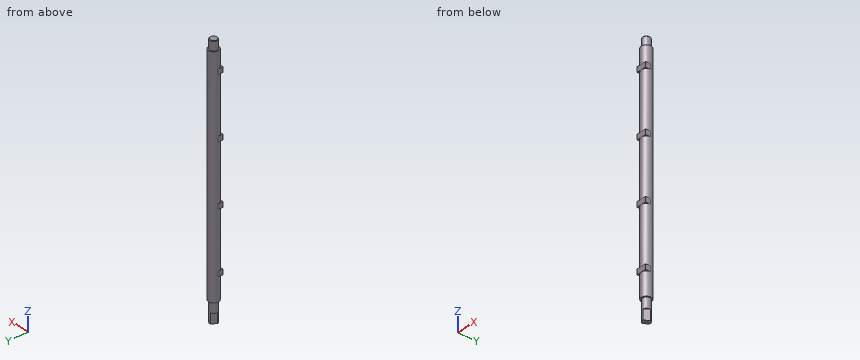
Autodesk Inventor part; units mm, degrees
ref_plane "工作平面1" through (0, 0, 45) normal (0, 0, -1) x (-1, 0, 0)
ref_plane "YZ Plane" through (0, 0, 0) normal (1, 0, 0) x (0, 1, 0)
ref_plane "XZ Plane" through (0, 0, 0) normal (0, 1, 0) x (-1, 0, 0)
sketch "草图1" plane through (0, 0, 0) normal (0, 0, 1) x (1, 0, 0)
  circle A0 centre (0, 0) radius 10
  dimension "d0" = 20
extrude "拉伸1" add sketch "草图1" along normal blind 447
sketch "草图2" plane through (0, 0, 447) normal (0, 0, 1) x (1, 0, 0)
  circle A0 centre (0, 0) radius 7.5
  dimension "d3" = 15
extrude "拉伸2" add sketch "草图2" along normal blind 18
chamfer "倒角1" distance 1 angle 45 1 edges at (-7.5, 0, 465)
sketch "草图3" plane through (0, 0, 0) normal (0, 0, -1) x (-1, 0, 0)
  circle A0 centre (0, 0) radius 7.5
  dimension "d9" = 15
extrude "拉伸3" add sketch "草图3" along normal blind 40
ref_plane "工作平面1" through (0, 0, 45) normal (0, 0, -1) x (-1, 0, 0)
sketch "草图4" plane through (0, 0, 45) normal (0, 0, -1) x (-1, 0, 0)
  circle A0 centre (0, 0) radius 10
  circle A1 centre (0, 0) radius 10
  line L0 (0, 10) -> (10, 10)
  line L1 (10, 0) -> (10, -10)
  line L2 (10, -10) -> (-10, -10)
  line L3 (-10, -10) -> (-10, 0)
  dimension "d13" = 20
  dimension "d14" = 20
  dimension "d15" = 10
  dimension "d16" = 10
extrude "拉伸4" add sketch "草图4" against normal blind 10 contours L1 L2 A0 | L2 L3 A0
pattern_linear "矩形阵列1" count 4 spacing 120 along (0, 0, 1) of "拉伸4"
sketch "草图5" plane through (0, 0, -40) normal (0, 0, -1) x (-1, 0, 0)
  circle A0 centre (0, 0) radius 7.5
  line L0 (7.2712, -1.8385) -> (1.0192, 7.4304)
  line L1 (-1.0192, -7.4304) -> (-7.2712, 1.8385)
  line L2 (-10, -10) -> (0, -10)
  dimension "d22" = 15
  dimension "d23" = 10
  dimension "d24" = 56
extrude "拉伸5" cut sketch "草图5" against normal blind 20 contours A0 L0 | L1 A0
properties part number "刀轴"
Source: CAD feature listing. Evaluate the final solid. Frame: model axes, mm. Give positions to 0.01 mm unless a question says otherwise; leave off trailing zeros. Order: outer loops, then holes, each group sorted by start corner. A loop starts at its lowest first (then second) coordinate and runs counter-clockwise, first axis right, second up. Notation, with made-up numbers: (76, -7.75) -> (105, -7.75) arc R12 ccw to (105, -2.75) -> close; hole circle Ø3 at (83.5, -1). An arc over 180 degrees is marked (long way). Use a Markdown table: item, result.
1) Contact query for flat-ended pins moving along their axis: P1, Ø6, axis at x = 4.5, z = 315.5, coming from the +Y side; P2, Ø8, axis at x = 6, z = 283.5, coming from the +Y side; P3, Ø3, axis at x = -3, y = -7.5, coming from the +Z side. Output: stop coordinate, or through.
Answer list:
| item | result |
|---|---|
| P1 | y = 9.89 |
| P2 | y = 9.8 |
| P3 | z = 464.92 |
2) Section query A-A, the plane z = 205.5. Return the cut outline in (x, y), then the cut area to 3 significant figures.
Answer list:
| item | result |
|---|---|
| outline | circle Ø20 at (0, 0) |
| area | 314 mm² |
3) Ray query, line 1 along Y through (x, z) = (6.75, 128.5); line 2 along Y through (x, z) = (1, 381). Return the intervals inside material, ascending. Write a range as [from, to].
Answer list:
| item | result |
|---|---|
| line 1 | [-7.38, 7.38] |
| line 2 | [-9.95, 9.95] |
